Source: three-view drawing plus pictorial views. Frame: mm from the lowest corner of the part. A direction names the side the tool comes from. Give positions to 0.01 mm unless a question says otherwise; leave off trailing zeros. Order: outer loops, then holes, each group sorted by start corner. A loop starts at its lowest first (then second) coordinate and runs counter-clockwise, first axis right, second up.
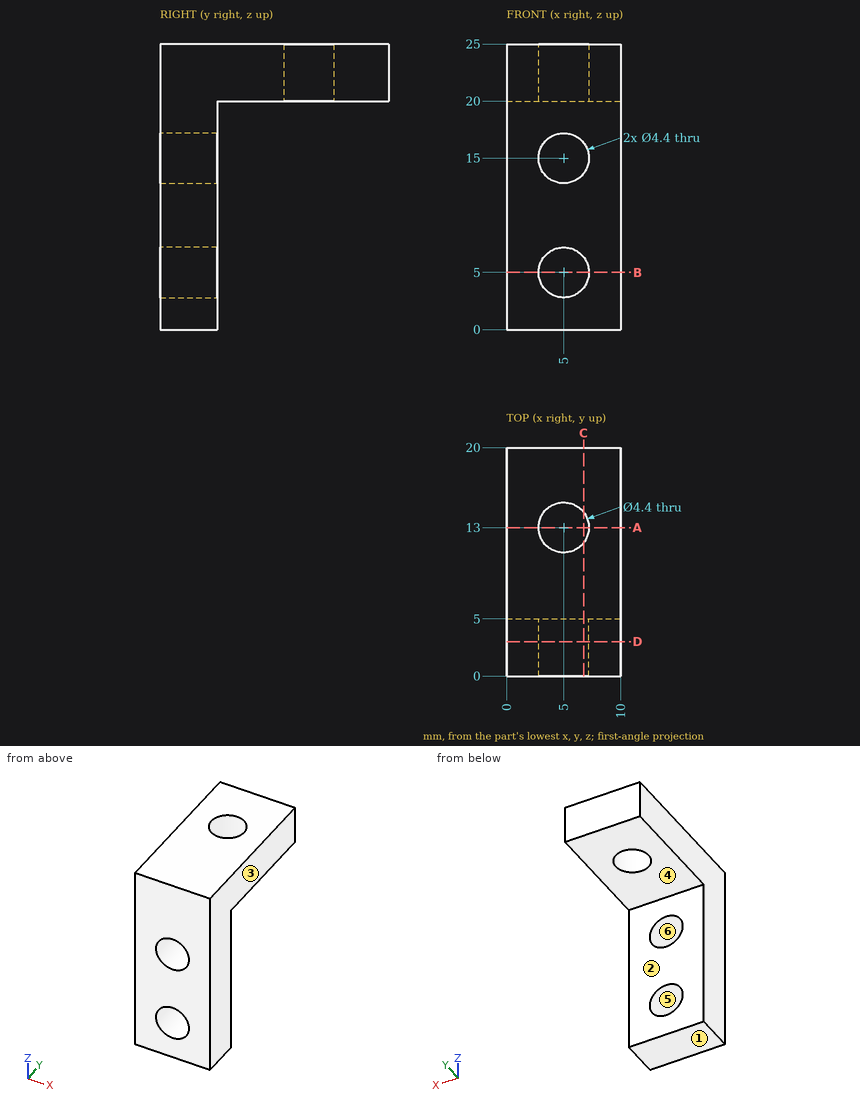
1) Section query B-B on z = 5. Output: boundary loops of the cut face in (x, y).
Checks:
outline: (0, 0) - (2.8, 0) - (2.8, 5) - (0, 5) - close; (7.2, 0) - (10, 0) - (10, 5) - (7.2, 5) - close
2) Section query A-A on y = 13. Output: boundary loops of the cut face in (x, z), and give its area (3 significant figures).
Checks:
outline: (0, 20) - (2.8, 20) - (2.8, 25) - (0, 25) - close; (7.2, 20) - (10, 20) - (10, 25) - (7.2, 25) - close
area: 28.0 mm2
3) First-contact query: pin 1 Ø5 at (x, y) = (5, 13) entering from -Z; pin 2 Ø3 at (x, z) = (4, 14.5) entering from +Y. Flat tips, straight axial feed; report the tip coordinate or a pass-through.
Checks:
pin 1: stops at z = 20
pin 2: stops at y = 5
4) Reachability of the marked faces 1 and 2 from +Z, -Z, +X, -X, +Y, -Y: full face, straight path, thin tool, end or side. Return the list, or none.
Checks:
face 1: -Z, +X, -X, +Y, -Y
face 2: -Z, +X, -X, +Y
5) Section query C-C on x = 6.75. Output: boundary loops of the cut face in (y, z), and give its area (3 significant figures).
Checks:
outline: (0, 0) - (5, 0) - (5, 3.67) - (0, 3.67) - close; (0, 6.33) - (5, 6.33) - (5, 13.67) - (0, 13.67) - close; (0, 16.33) - (5, 16.33) - (5, 20) - (11.67, 20) - (11.67, 25) - (0, 25) - close; (14.33, 20) - (20, 20) - (20, 25) - (14.33, 25) - close
area: 160 mm2
6) Section query D-D on y = 3. Output: boundary loops of the cut face in (x, z).
Checks:
outline: (0, 0) - (10, 0) - (10, 25) - (0, 25) - close; hole circle Ø4.4 at (5, 5); hole circle Ø4.4 at (5, 15)
7) Pull-direction query (X, two-part tool) for the marked faces 3, 4, 5 and 6; classes: +X half, -X half, draft (parallel to the pull), parting line (faces both ways), or undercut.
Checks:
face 3: +X half
face 4: draft
face 5: undercut
face 6: undercut
8) Ray query, L1, parallel to X at y = 2.55, z = 15; L2, parallel to Y at x = 5, z = 23; L3, parallel to Y at x = 6, z = 11. Return the intervals inside material, ascending.
Checks:
L1: x = 0 to 2.8, 7.2 to 10
L2: y = 0 to 10.8, 15.2 to 20
L3: y = 0 to 5
